Read the model definition and answer for the solid it produces. Units are mm, in the model's axes. A direction names the side the tool comes from. Give positions to 0.01 mm unless a question says otherwise; leave off trailing zeros. Order: outer loops, then holes, each group sorted by start corner. A loop starts at its lowest first (then second) coordinate and runs counter-clockwise, first axis right, second up.
```python
from build123d import *

# Parameters (mm, degrees)
F1_DEPTH = 25
F2_R     = 4.747339
F3_DEPTH = 25.001


with BuildPart() as f1:
    # F0 (on Top) → F1 (new body)
    with BuildSketch(Plane.XY):
        Polygon((-34.348406, -26.808511), (-23.736702, -26.808511), (-10.332447, -26.808511), (4.468086, -26.808511), (22.898939, -26.808511), (38.537234, -26.808511), (50.26596, -26.808511), (67.021281, -6.143617), (46.635643, -6.143617), (38.537234, -8.656915), (34.069151, -12.00798), (-3.07181, -12.00798), (-3.07181, -8.656915), (-62.273938, -8.656915), (-55.851065, -17.593086), (-46.635639, -24.295213), align=None)
    extrude(amount=F1_DEPTH)

    # F2 (on Top) → F3 (cut, through all)
    with BuildSketch(Plane.XY):
        with Locations((-23.736702, -15.079788)):
            Circle(F2_R)
    extrude(amount=F3_DEPTH, mode=Mode.SUBTRACT)


solid = f1.part
```
1) Consider L1, parallel to Y at x = -9.5, z = 9.5; L2, parallel to X at y = -13, z = 4; L3, parallel to X at y = -16.5, z = 17.75. Determine where each line is inside the solid, lowest interval first.
Final values:
L1: y = -26.81 to -8.66
L2: x = -59.15 to -28, -19.47 to 61.46
L3: x = -56.64 to -28.27, -19.21 to 58.62
2) The part is cut by section C-C on x = 9.5. Determine the outline of the cut face in (y, z).
Final values:
outline: (-26.81, 0) - (-12.01, 0) - (-12.01, 25) - (-26.81, 25) - close
3) The part is cut by section A-A on z = 5. Determine the outline of the cut face in (x, y), and give its area (3 significant figures).
Final values:
outline: (-62.27, -8.66) - (-55.85, -17.59) - (-46.64, -24.3) - (-34.35, -26.81) - (50.27, -26.81) - (67.02, -6.14) - (46.64, -6.14) - (38.54, -8.66) - (34.07, -12.01) - (-3.07, -12.01) - (-3.07, -8.66) - close; hole circle Ø9.49 at (-23.74, -15.08)
area: 1,880 mm2
4) The part is cut by section D-D on y = -22.75. Determine the outline of the cut face in (x, z), and give its area (3 significant figures).
Final values:
outline: (-48.76, 0) - (53.56, 0) - (53.56, 25) - (-48.76, 25) - close
area: 2,560 mm2
5) For a pull along X with two mould halves and no side action, classify faces 1 (the face through (16, -12.008, 12)), 2 (the face through (57, -6.144, 12)), 3 (the face through (-40.578, -25.534, 12.325)), 4 (the face through (-24.766, -19.714, 12.325)) as released by +X, released by -X, zero draft, split by the parting line, or undercut.
Final values:
face 1: undercut
face 2: zero draft
face 3: released by -X
face 4: undercut
6) Given pin 1 (1.5 mm diameter, centred on y = -22, z = 3, fed in from -X); pin 2 (5 mm diameter, centred on y = -9.5, z = 17, fed in from +X); pin 3 (2.5 mm diameter, centred on y = -11, z = 14, fed in from +X), each flat-ended and moving along its own axis, determine where each tip first touches the part or whether it passes through.
Final values:
pin 1: stops at x = -50.82
pin 2: stops at x = 66.33
pin 3: stops at x = 64.1
7) A tool of negligible diameter and unlimited length cuts with its end or side. For faces 5 (the face through (36.33, -10.31, 12.32)), 6 (the face through (-32, -8.657, 12)), 7 (the face through (7, -26.809, 12)), from which of +Z, -Z, +X, -X, +Y, -Y can it reach the whole face along a straight path? Write none if from no direction.
Final values:
face 5: +Z, -Z, +Y
face 6: +Z, -Z, -X, +Y
face 7: +Z, -Z, +X, -X, -Y
8) The part is cut by section B-B on x = -25.5. Determine the outline of the cut face in (y, z).
Final values:
outline: (-26.81, 0) - (-19.49, 0) - (-19.49, 25) - (-26.81, 25) - close; (-10.67, 0) - (-8.66, 0) - (-8.66, 25) - (-10.67, 25) - close
